```python
from build123d import *

# Parameters (mm, degrees)
SKETCH1_W           = 115
SKETCH1_H           = 65
SKETCH1_R           = 2.1
BOSS_EXTRUDE1_DEPTH = 22
SKETCH6_W           = 115
SKETCH6_H           = 65
SKETCH6_R           = 2.1
BOSS_EXTRUDE4_DEPTH = 3
SKETCH7_W           = 115
SKETCH7_H           = 65
BOSS_EXTRUDE5_DEPTH = 5
FILLET1_R           = 4
CUT_EXTRUDE1_REACH  = 32
SKETCH4_R           = 9.5
SKETCH4_R_2         = 3.5
CUT_EXTRUDE2_REACH  = 67


with BuildPart() as part:
    # Sketch1 → Boss-Extrude1 (new body)
    with BuildSketch(Plane(origin=(0, 0, 0), x_dir=(1, 0, 0), z_dir=(0, 1, 0))):
        with Locations((57.5, 32.5)):
            Rectangle(SKETCH1_W, SKETCH1_H)
        with Locations((108.9, 50.001511105)):
            Circle(SKETCH1_R, mode=Mode.SUBTRACT)
        with Locations((110.685057222, 6.404275632)):
            Circle(SKETCH1_R, mode=Mode.SUBTRACT)
        with Locations((7.785057222, 14.601511105)):
            Circle(SKETCH1_R, mode=Mode.SUBTRACT)
        with Locations((7.785057222, 55.601511105)):
            Circle(SKETCH1_R, mode=Mode.SUBTRACT)
        with BuildLine():
            Line((6.1, 47.31447682), (10.861715208, 47.31447682))
            ThreePointArc((10.861715208, 47.31447682), (12.346639448, 47.929552579), (12.961715208, 49.41447682))
            Line((12.961715208, 49.41447682), (12.961715208, 58.9))
            ThreePointArc((12.961715208, 58.9), (13.576790967, 60.38492424), (15.061715208, 61))
            Line((15.061715208, 61), (100.622896336, 61))
            ThreePointArc((100.622896336, 61), (102.107820577, 60.38492424), (102.722896336, 58.9))
            Line((102.722896336, 58.9), (102.722896336, 44.601511105))
            ThreePointArc((102.722896336, 44.601511105), (103.337972096, 43.116586864), (104.822896336, 42.501511105))
            Line((104.822896336, 42.501511105), (108.9, 42.501511105))
            ThreePointArc((108.9, 42.501511105), (110.38492424, 41.886435345), (111, 40.401511105))
            Line((111, 40.401511105), (111, 14.601511105))
            ThreePointArc((111, 14.601511105), (110.38492424, 13.116586864), (108.9, 12.501511105))
            Line((108.9, 12.501511105), (105.206624477, 12.501511105))
            ThreePointArc((105.206624477, 12.501511105), (103.721700237, 11.886435345), (103.106624477, 10.401511105))
            Line((103.106624477, 10.401511105), (103.106624477, 6.1))
            ThreePointArc((103.106624477, 6.1), (102.491548718, 4.61507576), (101.006624477, 4))
            Line((101.006624477, 4), (18.206624477, 4))
            ThreePointArc((18.206624477, 4), (16.721700237, 4.61507576), (16.106624477, 6.1))
            Line((16.106624477, 6.1), (16.106624477, 19.183092127))
            ThreePointArc((16.106624477, 19.183092127), (15.491548718, 20.668016368), (14.006624477, 21.283092127))
            Line((14.006624477, 21.283092127), (6.1, 21.283092127))
            ThreePointArc((6.1, 21.283092127), (4.61507576, 21.898167887), (4, 23.383092127))
            Line((4, 23.383092127), (4, 45.21447682))
            ThreePointArc((4, 45.21447682), (4.61507576, 46.69940106), (6.1, 47.31447682))
        make_face(mode=Mode.SUBTRACT)
    extrude(amount=BOSS_EXTRUDE1_DEPTH)

    # Sketch6 → Boss-Extrude4 (add)
    with BuildSketch(Plane.XZ):
        with Locations((57.5, -32.5)):
            Rectangle(SKETCH6_W, SKETCH6_H)
        with Locations((7.785057222, -14.601511105)):
            Circle(SKETCH6_R, mode=Mode.SUBTRACT)
        with Locations((110.685057222, -6.404275632)):
            Circle(SKETCH6_R, mode=Mode.SUBTRACT)
        with Locations((108.9, -50.001511105)):
            Circle(SKETCH6_R, mode=Mode.SUBTRACT)
        with Locations((7.785057222, -55.601511105)):
            Circle(SKETCH6_R, mode=Mode.SUBTRACT)
    extrude(amount=BOSS_EXTRUDE4_DEPTH)

    # Sketch7 → Boss-Extrude5 (add)
    with BuildSketch(Plane(origin=(0, 22, 0), x_dir=(1, 0, 0), z_dir=(0, 1, 0))):
        with Locations((57.5, 32.5)):
            Rectangle(SKETCH7_W, SKETCH7_H)
    extrude(amount=BOSS_EXTRUDE5_DEPTH)

    # Fillet1
    fillet1_edges = [part.edges().sort_by_distance(p)[0] for p in [
        (0, 12, -65),
        (115, 12, -65),
        (115, 12, 0),
        (0, 12, 0),
    ]]
    fillet(fillet1_edges, radius=FILLET1_R)

    # Sketch4 → Cut-Extrude1 (cut, up to next)
    with BuildSketch(Plane(origin=(0, 27, 0), x_dir=(1, 0, 0), z_dir=(0, 1, 0)), mode=Mode.PRIVATE) as cut_extrude1_sk1:
        with Locations((33, 46.5)):
            Circle(SKETCH4_R)
    cut_extrude1_tool1 = extrude(cut_extrude1_sk1.sketch, amount=-CUT_EXTRUDE1_REACH, mode=Mode.PRIVATE) & part.part
    add(cut_extrude1_tool1.solids().sort_by_distance((33, 27, -46.5))[0], mode=Mode.SUBTRACT)
    # Sketch4 → Cut-Extrude1 (cut, up to next)
    with BuildSketch(Plane(origin=(0, 27, 0), x_dir=(1, 0, 0), z_dir=(0, 1, 0)), mode=Mode.PRIVATE) as cut_extrude1_sk2:
        with Locations((33, 18.5)):
            Circle(SKETCH4_R)
    cut_extrude1_tool2 = extrude(cut_extrude1_sk2.sketch, amount=-CUT_EXTRUDE1_REACH, mode=Mode.PRIVATE) & part.part
    add(cut_extrude1_tool2.solids().sort_by_distance((33, 27, -18.5))[0], mode=Mode.SUBTRACT)
    # Sketch4 → Cut-Extrude1 (cut, up to next)
    with BuildSketch(Plane(origin=(0, 27, 0), x_dir=(1, 0, 0), z_dir=(0, 1, 0)), mode=Mode.PRIVATE) as cut_extrude1_sk3:
        with Locations((61, 46.5)):
            Circle(SKETCH4_R)
    cut_extrude1_tool3 = extrude(cut_extrude1_sk3.sketch, amount=-CUT_EXTRUDE1_REACH, mode=Mode.PRIVATE) & part.part
    add(cut_extrude1_tool3.solids().sort_by_distance((61, 27, -46.5))[0], mode=Mode.SUBTRACT)
    # Sketch4 → Cut-Extrude1 (cut, up to next)
    with BuildSketch(Plane(origin=(0, 27, 0), x_dir=(1, 0, 0), z_dir=(0, 1, 0)), mode=Mode.PRIVATE) as cut_extrude1_sk4:
        with Locations((89, 46.5)):
            Circle(SKETCH4_R)
    cut_extrude1_tool4 = extrude(cut_extrude1_sk4.sketch, amount=-CUT_EXTRUDE1_REACH, mode=Mode.PRIVATE) & part.part
    add(cut_extrude1_tool4.solids().sort_by_distance((89, 27, -46.5))[0], mode=Mode.SUBTRACT)
    # Sketch4 → Cut-Extrude1 (cut, up to next)
    with BuildSketch(Plane(origin=(0, 27, 0), x_dir=(1, 0, 0), z_dir=(0, 1, 0)), mode=Mode.PRIVATE) as cut_extrude1_sk5:
        with Locations((61, 18.5)):
            Circle(SKETCH4_R)
    cut_extrude1_tool5 = extrude(cut_extrude1_sk5.sketch, amount=-CUT_EXTRUDE1_REACH, mode=Mode.PRIVATE) & part.part
    add(cut_extrude1_tool5.solids().sort_by_distance((61, 27, -18.5))[0], mode=Mode.SUBTRACT)
    # Sketch4 → Cut-Extrude1 (cut, up to next)
    with BuildSketch(Plane(origin=(0, 27, 0), x_dir=(1, 0, 0), z_dir=(0, 1, 0)), mode=Mode.PRIVATE) as cut_extrude1_sk6:
        with Locations((89, 18.5)):
            Circle(SKETCH4_R)
    cut_extrude1_tool6 = extrude(cut_extrude1_sk6.sketch, amount=-CUT_EXTRUDE1_REACH, mode=Mode.PRIVATE) & part.part
    add(cut_extrude1_tool6.solids().sort_by_distance((89, 27, -18.5))[0], mode=Mode.SUBTRACT)
    # Sketch4 → Cut-Extrude1 (cut, up to next)
    with BuildSketch(Plane(origin=(0, 27, 0), x_dir=(1, 0, 0), z_dir=(0, 1, 0)), mode=Mode.PRIVATE) as cut_extrude1_sk7:
        with Locations((13, 32.5)):
            Circle(SKETCH4_R_2)
    cut_extrude1_tool7 = extrude(cut_extrude1_sk7.sketch, amount=-CUT_EXTRUDE1_REACH, mode=Mode.PRIVATE) & part.part
    add(cut_extrude1_tool7.solids().sort_by_distance((13, 27, -32.5))[0], mode=Mode.SUBTRACT)

    # Sketch5 → Cut-Extrude2 (cut, up to next)
    with BuildSketch(Plane.XY, mode=Mode.PRIVATE) as cut_extrude2_sk1:
        with BuildLine():
            Line((62.75, 7.055), (69.25, 7.055))
            ThreePointArc((69.25, 7.055), (71.45, 4.855), (69.25, 2.655))
            Line((69.25, 2.655), (62.75, 2.655))
            ThreePointArc((62.75, 2.655), (60.55, 4.855), (62.75, 7.055))
        make_face()
    cut_extrude2_tool1 = extrude(cut_extrude2_sk1.sketch, amount=-CUT_EXTRUDE2_REACH, mode=Mode.PRIVATE) & part.part
    add(cut_extrude2_tool1.solids().sort_by_distance((66, 4.855, 0))[0], mode=Mode.SUBTRACT)


solid = part.part
```
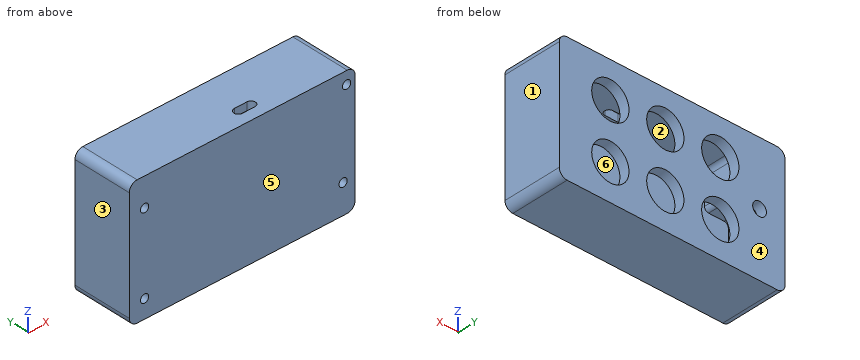
Check sheet for the modelled part. Datum: model origin and axes. Units: mm. Face numbers are marked on the shaded views. A direction names the side the tool comes from. Round coordinates to 2 decimals unless told otherwise and drop trailing zeros. Order: outer loops, then holes, each group sorted by start corner. A loop starts at its lowest first (then second) coordinate and runs counter-clockwise, first axis right, second up.
1) Section check C-C (x = 33). Record the boundary of the cut face in (y, z), and give its area (3 significant figures).
2) Tool access check on the marked faces 5 and 6. Record the directions out of +Z, -Z, +X, -X, +Y, -Y that give a thin tool (end or side, any length) a straight path to the whole face; none if there is none.
3) Scan lines: line 1 (X direction, y = 25.35, z = -18.5); line 2 (Z direction, x = 53, y = 2); line 3 (Z direction, x = 33, y = 25.45). Record each from-to range of solid material in increasing order.
4) Section check D-D (z = -32.5). Record the boundary of the cut face in (x, y).
5) Mould release check, pull along X, two halves, no side actions. Record for the marked faces 1, 2, 3 and 4: +X half, -X half, draft (parallel to the pull), parting line (faces both ways), or undercut.
6) Go/stop test with flat-tipped pins: pin 1 Ø4.5 at (x, z) = (110.5, -5.5) entering from -Y; pin 2 Ø5 at (x, z) = (39.5, -46) entering from +Y. Record where each tip stops, or that it passes through.
7) Section check B-B (y = 23.5). Record the boundary of the cut face in (x, z).
8) Section check A-A (x = 49). Record the boundary of the cut face in (y, z), and give its area (3 significant figures).
Result:
1. outline: (-3, -65) - (27, -65) - (27, -56) - (22, -56) - (22, -61) - (0, -61) - (0, -4) - (22, -4) - (22, -9) - (27, -9) - (27, 0) - (-3, 0) - close; (22, -37) - (27, -37) - (27, -28) - (22, -28) - close
1. area: 506 mm2
2. face 5: +Z, -Z, +X, -X, -Y
2. face 6: none
3. line 1: x = 0 to 23.5, 42.5 to 51.5, 70.5 to 79.5, 98.5 to 115
3. line 2: z = -65 to -61, -4 to 0
3. line 3: z = -65 to -56, -37 to -28, -9 to 0
4. outline: (0, -3) - (115, -3) - (115, 27) - (16.5, 27) - (16.5, 22) - (111, 22) - (111, 0) - (4, 0) - (4, 22) - (9.5, 22) - (9.5, 27) - (0, 27) - close
5. face 1: +X half
5. face 2: undercut
5. face 3: -X half
5. face 4: draft
6. pin 1: stops at y = -3
6. pin 2: stops at y = 0
7. outline: (0, -61) arc R4 ccw to (4, -65) - (111, -65) arc R4 ccw to (115, -61) - (115, -4) arc R4 ccw to (111, 0) - (4, 0) arc R4 ccw to (0, -4) - close; hole circle Ø7 at (13, -32.5); hole circle Ø19 at (33, -46.5); hole circle Ø19 at (33, -18.5); hole circle Ø19 at (61, -46.5); hole circle Ø19 at (61, -18.5); hole circle Ø19 at (89, -46.5); hole circle Ø19 at (89, -18.5)
8. outline: (-3, -65) - (27, -65) - (27, 0) - (-3, 0) - close; hole (0, -61) - (22, -61) - (22, -4) - (0, -4) - close
8. area: 696 mm2
